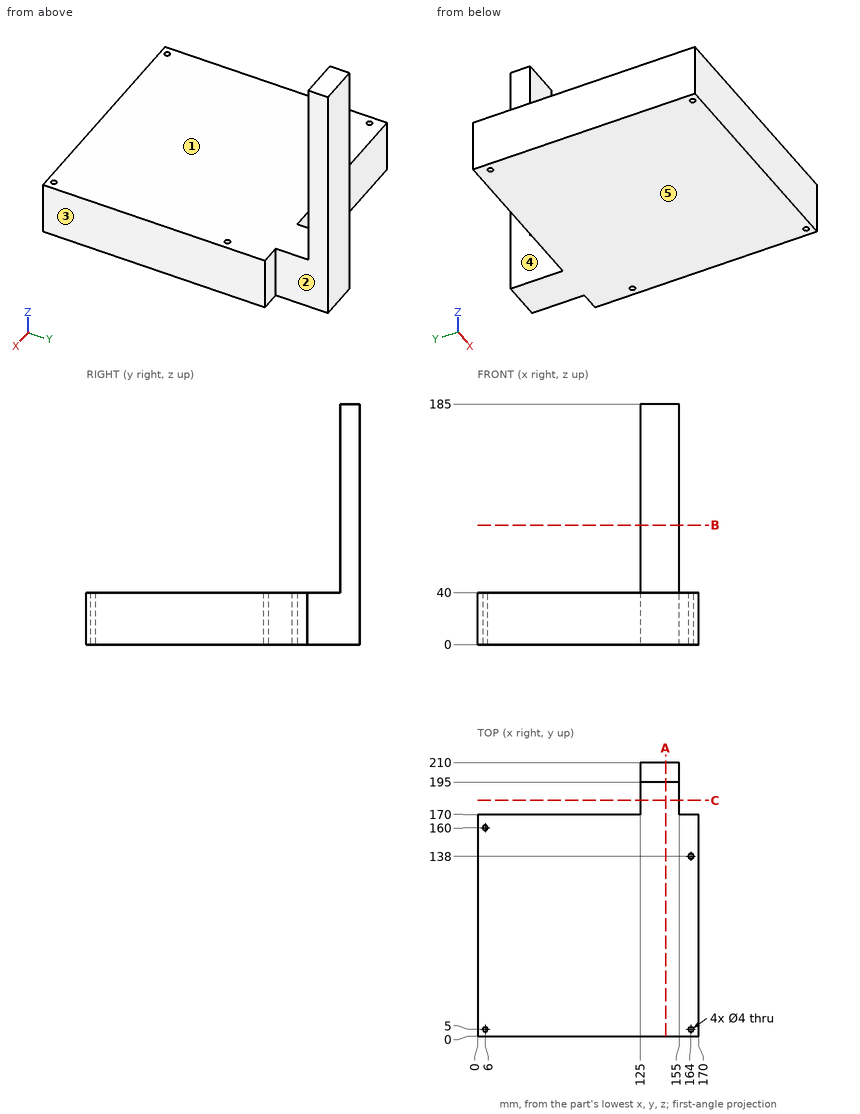
Here's the drawing with two shaded views (mm, measured from the low corner). I have some questions. A direction names the side the tool comes from. Coordinates: 2 decimals unless noted, no trailing zeros. Write each loop counter-clockwise with the first axis right and the second up, starting at its lowest first coordinate (ties: lowest second). Pieces come first, ordered by that corner, then holes.
Item 1: I want a section at C-C on y = 181. Write out the boundary of the cut face in (x, z).
Item 2: On a 3-axis mill with a long thin cutter (end or side, diameter ignored), from which of +Z, -Z, +X, -X, +Y, -Y can I reach the whole of each face in a straight line? I mean the marked faces 1, 2, 3, 4 and 5. Say none if no direction works.
Item 3: Will these pins go through, and if not, where does the flat tip stop? pin 1 (7.5 mm diameter, centred on x = 160.5, z = 11, fed in from +Y); pin 2 (2.5 mm diameter, centred on x = 6, y = 5, fed in from -Z) (1 decimal); pin 3 (12 mm diameter, centred on y = 192.5, z = 66.5, fed in from -X); pin 4 (6.5 mm diameter, centred on x = 6, y = 160, fed in from +Z).
Item 4: If I drill on line 1 (Y direction, x = 6, z = 19); line 2 (Y direction, x = 164, z = 29.5); line 3 (X direction, y = 138, z = 26), over which ranges is the centre line in solid material (lowest first)?
Item 5: I want a section at B-B on z = 92. Write out the boundary of the cut face in (x, y), and give its area (3 significant figures).
Item 6: I want a section at A-A on x = 144.5. Write out the boundary of the cut face in (y, z), and give its area (3 significant figures).
Findings below:
1. outline: (125, 0) - (155, 0) - (155, 40) - (125, 40) - close
2. face 1: +Z, +X, -X, -Y
2. face 2: +Z, -Z, +X, +Y
2. face 3: +Z, -Z, +X, +Y, -Y
2. face 4: +Z, -Z, -X, +Y
2. face 5: -Z, +X, -X, +Y, -Y
3. pin 1: stops at y = 170
3. pin 2: passes through
3. pin 3: stops at x = 125
3. pin 4: stops at z = 40
4. line 1: y = 0 to 3, 7 to 158, 162 to 170
4. line 2: y = 0 to 3, 7 to 136, 140 to 170
4. line 3: x = 0 to 162, 166 to 170
5. outline: (125, 195) - (155, 195) - (155, 210) - (125, 210) - close
5. area: 450 mm2
6. outline: (0, 0) - (210, 0) - (210, 185) - (195, 185) - (195, 40) - (0, 40) - close
6. area: 10,600 mm2
